Verification items for the finished model (mm, model axes). Face numbers are marked on the shaded views. Give positions to 0.01 mm unless a question says otherwise; leave off trailing zeros. Order: outer loops, then holes, each group sorted by start corner. A loop starts at its lowest first (then second) coordinate and runs counter-clockwise, first axis right, second up.
(1) Sectioned sample at B-B on z = 34.5. Record the cut outline in (x, y).
(2) Scan lines: L1, parallel to Y at x = 33, z = 3; L2, parallel to Z at x = -37, y = 1; L3, parallel to X at y = -176.5, z = 42.5. Record each from-to range of solid material in increasing order.
(3) Sectioned sample at A-A on y = -154.5. Record the cut outline in (x, z).
(4) Gauge pin test, flat ends, axial feed: pin 1 (5 mm diameter, centred on x = -37.5, z = 22, fed in from +Y); pin 2 (15.5 mm diameter, centred on y = -357, z = 32.5, fed in from +X); pin 3 (6.5 mm diameter, centred on x = -1, z = 49, fed in from -Y); pin 4 (4 mm diameter, centred on x = 16, y = 1.5, fed in from +Z). Record the tip position at first contact, or that the pin passes through.
(5) Mould release check, pull along X, two halves, no side actions. Record for the marked faces 1, 2 and 3: pulls with the +X half, pulls with the -X half, needs draft (parallel to the pull), parting line crosses it, or undercut.
```python
from build123d import *

# Parameters (mm, degrees)
F0_W     = 55
F0_H     = 55
F1_DEPTH = 590
F2_W     = 15
F2_H     = 45
F2_R     = 3
F2_W_2   = 55
F3_DEPTH = 5
F4_W     = 15
F4_H     = 45
F4_R     = 3
F4_W_2   = 55
F5_DEPTH = 5
F6_R     = 2


with BuildPart() as f1:
    # F0 (on Front) → F1 (new body)
    with BuildSketch(Plane.XZ):
        with Locations((0, 27.5)):
            Rectangle(F0_W, F0_H)
    extrude(amount=F1_DEPTH)

    # F2 (on face) → F3 (join)
    with BuildSketch(Plane(origin=(0, 0, 0), x_dir=(-1, 0, 0), z_dir=(0, 1, 0))):
        with Locations((-35, 22.5)):
            Rectangle(F2_W, F2_H)
        with Locations((-37.5, 22)):
            Circle(F2_R, mode=Mode.SUBTRACT)
        with Locations((0, 22.5)):
            Rectangle(F2_W_2, F2_H)
        with Locations((35, 22.5)):
            Rectangle(F2_W, F2_H)
        with Locations((37.5, 22)):
            Circle(F2_R, mode=Mode.SUBTRACT)
    extrude(amount=F3_DEPTH)

    # F4 (on face) → F5 (join)
    with BuildSketch(Plane.XZ.offset(590)):
        with Locations((-35, 22.5)):
            Rectangle(F4_W, F4_H)
        with Locations((-37.5, 22)):
            Circle(F4_R, mode=Mode.SUBTRACT)
        with Locations((0, 22.5)):
            Rectangle(F4_W_2, F4_H)
        with Locations((35, 22.5)):
            Rectangle(F4_W, F4_H)
        with Locations((37.5, 22)):
            Circle(F4_R, mode=Mode.SUBTRACT)
    extrude(amount=F5_DEPTH)

    # F6
    f6_edges = [f1.edges().sort_by_distance(p)[0] for p in [
        (27.5, -295, 55),
        (-27.5, -295, 55),
        (0, 0, 55),
        (0, -590, 55),
        (-27.5, -295, 0),
        (27.5, -295, 0),
    ]]
    fillet(f6_edges, radius=F6_R)


solid = f1.part
```
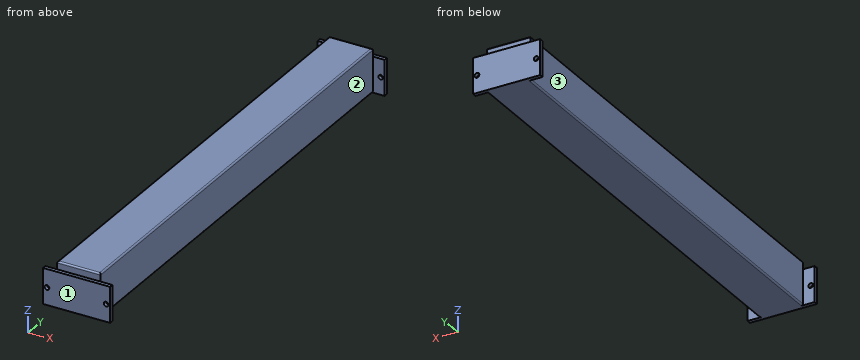
Ans:
1. outline: (-42.5, -595) - (42.5, -595) - (42.5, -590) - (27.5, -590) - (27.5, 0) - (42.5, 0) - (42.5, 5) - (-42.5, 5) - (-42.5, 0) - (-27.5, 0) - (-27.5, -590) - (-42.5, -590) - close
2. L1: y = -595 to -590, 0 to 5
2. L2: z = 0 to 19.04, 24.96 to 45
2. L3: x = -27.5 to 27.5
3. outline: (-27.5, 2) arc R2 ccw to (-25.5, 0) - (25.5, 0) arc R2 ccw to (27.5, 2) - (27.5, 53) arc R2 ccw to (25.5, 55) - (-25.5, 55) arc R2 ccw to (-27.5, 53) - close
4. pin 1: passes through
4. pin 2: stops at x = 27.5
4. pin 3: stops at y = -590
4. pin 4: stops at z = 54.32
5. face 1: needs draft
5. face 2: pulls with the +X half
5. face 3: pulls with the -X half
